```python
from build123d import *

# Parameters (mm, degrees)
SKETCH_3_R      = 2.5
EXTRUDE_3_DEPTH = 5


with BuildPart() as part:
    # 草圖3 → 填料-伸長3 (new body)
    with BuildSketch(Plane(origin=(0, 0, 0), x_dir=(0, 0, -1), z_dir=(1, 0, 0))):
        with BuildLine():
            Line((0, -9), (-34.64, -9))
            ThreePointArc((-34.64, -9), (-25.64, 0), (-34.64, 9))
            Line((-34.64, 9), (0, 9))
            ThreePointArc((0, 9), (9, 0), (0, -9))
        make_face()
        Circle(SKETCH_3_R, mode=Mode.SUBTRACT)
    extrude(amount=EXTRUDE_3_DEPTH)


solid = part.part
```
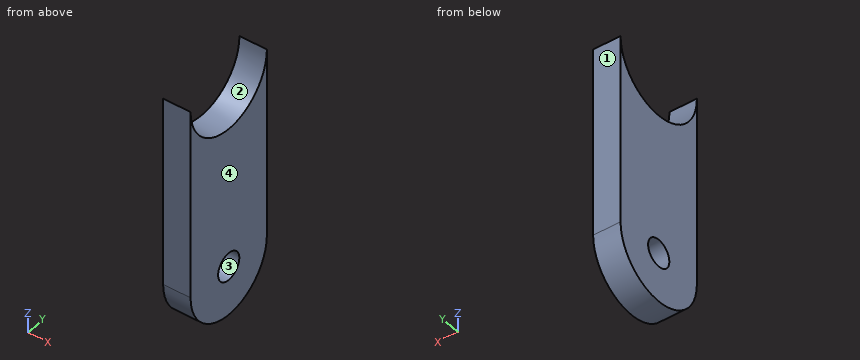
For this review, take the finished solid that the model builds, in its own axes (mm). Face numbers are marked on the shaded views. Coordinates: 2 decimals unless noted, no trailing zeros. Order: outer loops, then holes, each group sorted by start corner. A loop starts at its lowest first (then second) coordinate and runs counter-clockwise, first axis right, second up. Notation, with made-up numbers: (48.5, 11) -> (52.5, 11) arc R34 ccw to (52.5, 43) -> close; hole circle Ø10 at (-40, -33). An arc over 180 degrees is marked (long way). Answer as CSV lines item,"result".
Q1. Clearance check with a flat-ended pin moving along its axis: pin 1 Ø1.5 at (x, y) = (1, 3.5) entering from +Z. State where the tip first meets the part, or that it passes through.
Model answer:
pin 1,"stops at z = 26.71"
Q2. Wall thickness on line 1 along Z through (x, y) = (3.1, -0.5); line 2 along Z through (x, y) = (3.6, -1.75); line 3 along Y through (x, z) = (3.95, 30): over which ranges is each line inside the solid? List them lowest first. Write a range as [from, to].
Model answer:
line 1,"z = [-8.99, -2.45], [2.45, 25.65]"
line 2,"z = [-8.83, -1.79], [1.79, 25.81]"
line 3,"y = [-9, -7.71], [7.71, 9]"
Q3. We need section A-A (y = 0). State the section outline as (x, z) points.
Model answer:
outline,"(0, -9) -> (5, -9) -> (5, -2.5) -> (0, -2.5) -> close; (0, 2.5) -> (5, 2.5) -> (5, 25.64) -> (0, 25.64) -> close"
Q4. We need section D-D (y = 3). State the section outline as (x, z) points, plus the area to 3 significant figures.
Model answer:
outline,"(0, -8.49) -> (5, -8.49) -> (5, 26.15) -> (0, 26.15) -> close"
area,"173 mm2"
Q5. We need section C-C (x = 0.45). State the section outline as (y, z) points, plus the area to 3 significant figures.
Model answer:
outline,"(-9, 0) arc R9 ccw to (9, 0) -> (9, 34.64) arc R9 cw to (-9, 34.64) -> close; hole circle Ø5 at (0, 0)"
area,"604 mm2"
Q6. Draft analysis for pull direction Y (two halves, no side actions). For the marked faces 1, 2, 3 and 4, state which applies: released by +Y, released by -Y, zero draft, split by the parting line, or undercut.
Model answer:
face 1,"released by +Y"
face 2,"undercut"
face 3,"undercut"
face 4,"zero draft"
Q7. We need section B-B (z = 2). State the section outline as (x, y) points, plus the area to 3 significant figures.
Model answer:
outline,"(0, -9) -> (5, -9) -> (5, -1.5) -> (0, -1.5) -> close; (0, 1.5) -> (5, 1.5) -> (5, 9) -> (0, 9) -> close"
area,"75.0 mm2"
